Drawing for the job (mm, zero at the part's lowest x, y, z). A direction names the side the tool comes from. Round coordinates to 2 decimals unless told otherwise and drop trailing zeros. Order: outer loops, then holes, each group sorted by start corner. A loop starts at its lowest first (then second) coordinate and runs counter-clockwise, first axis right, second up. Notation, with made-up numbers: (-11, -27.5) - (19, -27.5) arc R22 cw to (19, 4.5) - close; hole circle Ø7 at (-11, 62). An arc over 180 degrees is marked (long way). Put each result on its own line as item: value. Start each with the question number.
Item 1: Mould opens along X. For the marked faces 6, 7, 8 and 9 say: pulls with the +X half, pulls with the -X half, needs draft (parallel to the pull), parting line crosses it, or undercut.
Item 2: Which spindle directions (+Z, -Z, +X, -X, +Y, -Y) get a long thin tool onto all of the face, cutting with end or side? Do the marked faces 1, 2, 3, 4 and 5. Say none if no direction does.
Item 3: Probe probe 1 along X at (y, z) = (1.25, 41.5) (1 decimal); probe 2 along X at (y, z) = (2, 71.5) (1 decimal); probe 3 along Y at (x, z) = (10.5, 87). List the from-to ranges inside material, lowest first.
Item 4: Saw through at A-A on z = 24. List the corners of the cut face in (x, y) (1 decimal), plus the area to 3 significant figures.
Item 5: Saw through at C-C on x = 16. List the corners of the cut face in (y, z).
Item 6: Saw through at B-B on x = 34. List the corners of the cut face in (y, z), plus the area to 3 significant figures.
Item 7: Pin check, flat tips, straight feed: pin 1 Ø12 at (x, z) = (34.5, 61) entering from +Y; pin 2 Ø3 at (x, z) = (17.5, 83) entering from +Y; pin 3 Ø7.5 at (x, z) = (9.5, 32.5) entering from -Y. Stop position of each tip, or through.
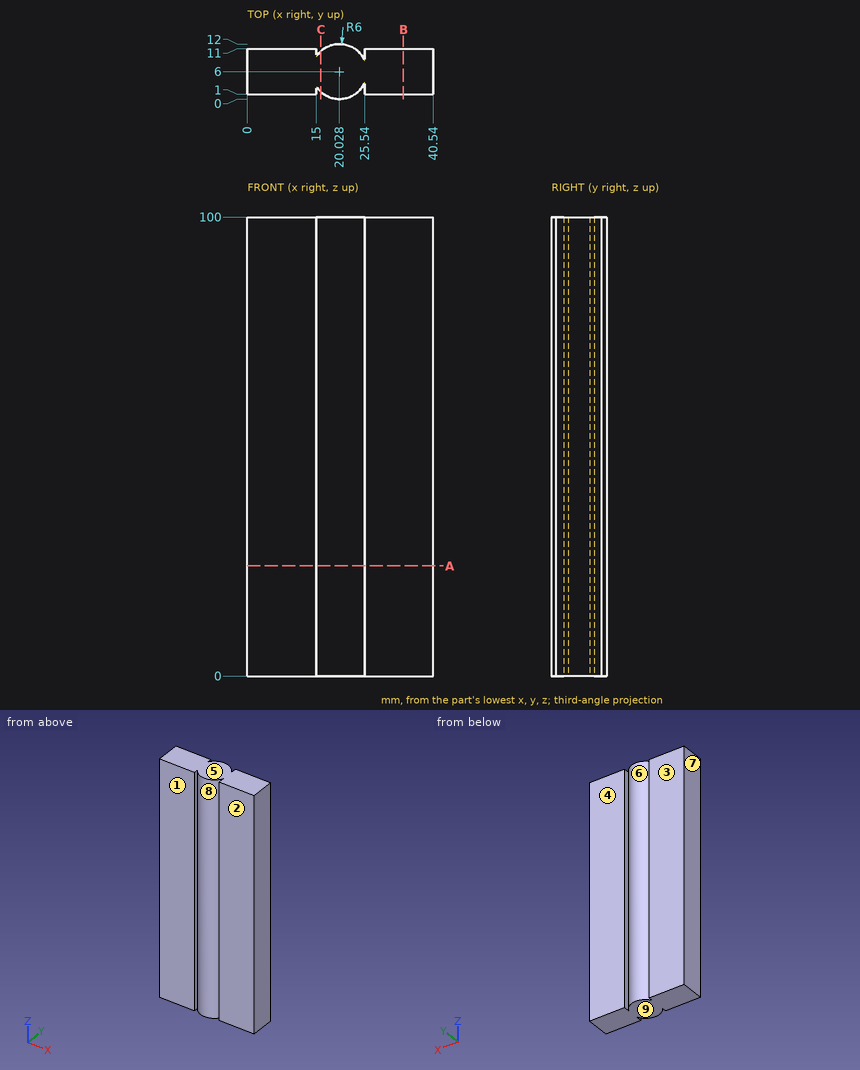
Results found:
1. face 6: undercut
1. face 7: pulls with the -X half
1. face 8: undercut
1. face 9: needs draft
2. face 1: +Z, -Z, -X, -Y
2. face 2: +Z, -Z, +X, -Y
2. face 3: +Z, -Z, -X, +Y
2. face 4: +Z, -Z, +X, +Y
2. face 5: +Z, +X, -X, +Y, -Y
3. probe 1: x = 0 to 15, 16.4 to 23.7, 25.5 to 40.5
3. probe 2: x = 0 to 15, 15.6 to 24.5, 25.5 to 40.5
3. probe 3: y = 1 to 11
4. outline: (0, 1) - (15, 1) - (15, 2.7) arc R6 ccw to (25.5, 3.6) - (25.5, 1) - (40.5, 1) - (40.5, 11) - (25.5, 11) - (25.5, 8.4) arc R6 ccw to (15, 9.3) - (15, 11) - (0, 11) - close
4. area: 407 mm²
5. outline: (1.55, 0) - (10.45, 0) - (10.45, 100) - (1.55, 100) - close
6. outline: (1, 0) - (11, 0) - (11, 100) - (1, 100) - close
6. area: 1,000 mm²
7. pin 1: stops at y = 11
7. pin 2: stops at y = 11.91
7. pin 3: stops at y = 1
